Could you check a few things on this model? Use its own coordinates, in mm. A direction names the side the tool comes from. Coordinates: 2 decimals unless noted, no trailing zeros. Loops run counter-clockwise (first coordinate to the right, second up) from the corner with the lowest first, then second, coordinate; pieces in that order, holes last. Notation, with made-up numbers: (-2, 32.25) -> (12, 32.25) arc R22 ccw to (12, 54.25) -> close; hole circle Ø10 at (78.25, 19). An arc over 180 degrees is marked (long way). One line per question, with ' | ' between items.
```python
from build123d import *

# Parameters (mm, degrees)
SKETCH1_W           = 10
SKETCH1_H           = 7.5
SKETCH1_R           = 1
BOSS_EXTRUDE1_DEPTH = 44
SKETCH1_3_R         = 1
CUT_EXTRUDE1_DEPTH  = 5
SKETCH2_R           = 1
CUT_EXTRUDE2_DEPTH  = 5


with BuildPart() as part:
    # Sketch1 → Boss-Extrude1 (new body)
    with BuildSketch(Plane(origin=(0, 0, 0), x_dir=(0, 0, -1), z_dir=(1, 0, 0))):
        with Locations((5, 11.25)):
            Rectangle(SKETCH1_W, SKETCH1_H)
        with Locations((3, 12)):
            Circle(SKETCH1_R, mode=Mode.SUBTRACT)
        with Locations((3, 12)):
            Circle(SKETCH1_R)
        with Locations((15, 11.25)):
            Rectangle(SKETCH1_W, SKETCH1_H)
        with Locations((17, 12)):
            Circle(SKETCH1_R, mode=Mode.SUBTRACT)
        with Locations((17, 12)):
            Circle(SKETCH1_R)
        with Locations((15, 3.75)):
            Rectangle(SKETCH1_W, SKETCH1_H)
        with Locations((17, 3)):
            Circle(SKETCH1_R, mode=Mode.SUBTRACT)
        with Locations((17, 3)):
            Circle(SKETCH1_R)
        with Locations((5, 3.75)):
            Rectangle(SKETCH1_W, SKETCH1_H)
        with Locations((3, 3)):
            Circle(SKETCH1_R, mode=Mode.SUBTRACT)
        with Locations((3, 3)):
            Circle(SKETCH1_R)
    extrude(amount=-BOSS_EXTRUDE1_DEPTH)

    # Sketch1_3 → Cut-Extrude1 (cut)
    with BuildSketch(Plane(origin=(0, 0, 0), x_dir=(0, 0, -1), z_dir=(1, 0, 0))):
        with Locations((3, 12)):
            Circle(SKETCH1_3_R)
        with Locations((17, 12)):
            Circle(SKETCH1_3_R)
        with Locations((17, 3)):
            Circle(SKETCH1_3_R)
        with Locations((3, 3)):
            Circle(SKETCH1_3_R)
    extrude(amount=-CUT_EXTRUDE1_DEPTH, mode=Mode.SUBTRACT)

    # Sketch2 → Cut-Extrude2 (cut)
    with BuildSketch(Plane.ZY.offset(44)):
        with Locations((-17, 12)):
            Circle(SKETCH2_R)
        with Locations((-3, 12)):
            Circle(SKETCH2_R)
        with Locations((-3, 3)):
            Circle(SKETCH2_R)
        with Locations((-17, 3)):
            Circle(SKETCH2_R)
    extrude(amount=-CUT_EXTRUDE2_DEPTH, mode=Mode.SUBTRACT)


solid = part.part
```
Q1. Imagine slicing it at B-B on y = 12. Write out the boundary of the cut face in (x, z), plus the area to 3 significant figures.
Values follow:
outline: (-44, -20) -> (0, -20) -> (0, -18) -> (-5, -18) -> (-5, -16) -> (0, -16) -> (0, -4) -> (-5, -4) -> (-5, -2) -> (0, -2) -> (0, 0) -> (-44, 0) -> (-44, -2) -> (-39, -2) -> (-39, -4) -> (-44, -4) -> (-44, -16) -> (-39, -16) -> (-39, -18) -> (-44, -18) -> close | area: 840 mm2
Q2. For pin 1 (0.6 mm diameter, centred on y = 3, z = -17, fed in from +X); pin 2 (0.6 mm diameter, centred on y = 3, z = -2.5, fed in from -X), each with a flat end and sliding along its axis, tell me the tip position at first contact or that it passes through.
Values follow:
pin 1: stops at x = -5 | pin 2: stops at x = -39
Q3. For faces 1 (the face through (-22, 7, -20)), 2 (the face through (-39, 3, -3)), 3 (the face through (-5, 12, -3)), which set-ups out of +Z, -Z, +X, -X, +Y, -Y let a thin tool reach every point of the face, with its end or its side?
Values follow:
face 1: -Z, +X, -X, +Y, -Y | face 2: -X | face 3: +X
Q4. Please list where this line runs through material, in increasing order: L1, parallel to Y at x = -42.6, z = -17. Write a range as [from, to].
Values follow:
L1: y = [0, 2], [4, 11], [13, 15]
Q5. Imagine slicing it at A-A on z = -17. Write out the boundary of the cut face in (x, y), plus the area to 3 significant figures.
Values follow:
outline: (-44, 0) -> (0, 0) -> (0, 2) -> (-5, 2) -> (-5, 4) -> (0, 4) -> (0, 11) -> (-5, 11) -> (-5, 13) -> (0, 13) -> (0, 15) -> (-44, 15) -> (-44, 13) -> (-39, 13) -> (-39, 11) -> (-44, 11) -> (-44, 4) -> (-39, 4) -> (-39, 2) -> (-44, 2) -> close | area: 620 mm2
Q6. We'd pull the mould along Y, two halves only. Please class faces 4 (the face through (-42, 3, -16)), 5 (the face through (-44, 8, -10)), 6 (the face through (-22, 15, -10)), 7 (the face through (-5, 3, -3)): released by +Y, released by -Y, zero draft, split by the parting line, or undercut.
Values follow:
face 4: undercut | face 5: zero draft | face 6: released by +Y | face 7: undercut
